Part model, mm, in its own coordinate system. Face numbers are marked on the shaded views. A direction names the side the tool comes from. Give positions to 0.01 mm unless a question says otherwise; leave off trailing zeros. Order: outer loops, then holes, each group sorted by start corner. A loop starts at its lowest first (then second) coordinate and runs counter-clockwise, first axis right, second up. Notation, with made-up numbers: (64.25, 62.25) - (72.25, 62.25) arc R22 ccw to (72.25, 73.25) - close; hole circle Ø4 at (2, -11.75). An arc over 180 degrees is marked (long way). Use a Markdown table: item, result. Add a question column.
from build123d import *

# Parameters (mm, degrees)
F0_R     = 1.5
F1_DEPTH = 5


with BuildPart() as f1:
    # F0 (on Top) → F1 (new body)
    with BuildSketch(Plane.XY):
        with BuildLine():
            Line((0, 20.066716), (0, 0))
            Line((0, 0), (5, 0))
            Line((5, 0), (5, 15.066716))
            Line((5, 15.066716), (45, 15.066716))
            Line((45, 15.066716), (45, 2))
            ThreePointArc((45, 2), (45.585786, 0.585786), (47, 0))
            Line((47, 0), (48, 0))
            ThreePointArc((48, 0), (49.414214, 0.585786), (50, 2))
            Line((50, 2), (50, 20.066716))
            Line((50, 20.066716), (0, 20.066716))
        make_face()
        with Locations((2.913021, 17.143138)):
            Circle(F0_R, mode=Mode.SUBTRACT)
    extrude(amount=F1_DEPTH)


solid = f1.part
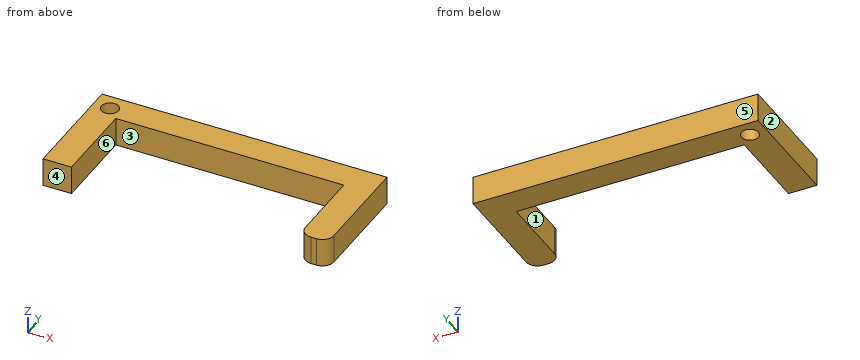
1. Drill centre lines: probe 1 along X at (y, z) = (11.25, 0.7); probe 2 along Y at (x, z) = (11.5, 4.8); probe 3 along Y at (x, z) = (4, 0.35). Where is each one in solid material? Low to high. Write a range as [from, to].
2. Cut at A-A (y = 3). Write the cut outline in (x, z), plus the area to 3 significant figures.
3. Mould opens along X. For the marked faces 1, 2, 3 and 4 say: released by +X, released by -X, zero draft, split by the parting line, or undercut.
4. Cut at B-B (z = 0.75). Write the cut outline in (x, y).
5. Cut at C-C (x = 33). Write the cut outline in (y, z), plus the area to 3 significant figures.
6. Tool access for the marked faces 5 and 6: list every direction of +Z, -Z, +X, -X, +Y, -Y with a clear straight run to the whole face (end or side of a thin tool).
Responses:
| question | item | result |
|---|---|---|
| 1 | probe 1 | x = [0, 5], [45, 50] |
| 1 | probe 2 | y = [15.07, 20.07] |
| 1 | probe 3 | y = [0, 16.11], [18.18, 20.07] |
| 2 | outline | (0, 0) - (5, 0) - (5, 5) - (0, 5) - close; (45, 0) - (50, 0) - (50, 5) - (45, 5) - close |
| 2 | area | 50.0 mm² |
| 3 | face 1 | undercut |
| 3 | face 2 | released by -X |
| 3 | face 3 | undercut |
| 3 | face 4 | zero draft |
| 4 | outline | (0, 0) - (5, 0) - (5, 15.07) - (45, 15.07) - (45, 2) arc R2 ccw to (47, 0) - (48, 0) arc R2 ccw to (50, 2) - (50, 20.07) - (0, 20.07) - close; hole circle Ø3 at (2.91, 17.14) |
| 5 | outline | (15.07, 0) - (20.07, 0) - (20.07, 5) - (15.07, 5) - close |
| 5 | area | 25.0 mm² |
| 6 | face 5 | +Z, -Z, +X, -X, +Y |
| 6 | face 6 | +Z, -Z, -Y |
